Input: part model. Units: mm. Frame: model coordinates. A direction names the side the tool comes from. Give positions to 0.01 mm unless a question says otherwise; leave off trailing zeros. Write each loop counter-clockwise with the first axis right and the second up, starting at its lowest first coordinate (ties: lowest second). Pieces come first, ordered by that corner, then holes. Notation, with made-up numbers: (-14, 88.5) -> (8, 88.5) arc R20 cw to (8, 105.5) -> close; hole circle Ø4 at (-25, 57.25). An arc over 180 degrees is marked (long way). Return JSON: item names as keys, results as strings. Group by question number.
Item 1: Section C-C, the plane y = 7. Return loops of the section in (x, z) (3 decimals).
Item 2: Pin query (flat end, axial travel): P1, Ø5, axis at x = 17.5, z = -1.5, coming from the -Y side; P2, Ø5, axis at x = 17.5, z = 7.5, coming from the +Y side. Return the tip coordinate at first contact, or that it passes through.
Item 3: Set-up query: faces 1 (the face through (11.4, 3.94, 3.93)), 2 (the face through (0, 8, -6)). Return all of +Z, -Z, +X, -X, +Y, -Y with unobstructed straight access to the full face (end or side cutting, diameter ignored); none if empty.
Item 4: Section B-B, the plane z = 1. Return loops of the section in (x, y).
Item 5: Section D-D, the plane x = -17.5. Return loops of the section in (y, z) (3 decimals).
Item 6: Mould query, pull axis X, two halves, no side actions, for faces 3 (the face through (22.5, 4, 0)), 4 (the face through (0, 4, -12.5)), 5 (the face through (-11.4, 3.94, -3.93)). Classes: released by +X, released by -X, zero draft, split by the parting line, or undercut.
Item 7: Section A-A, the plane z = 7.5. Return loops of the section in (x, y) (3 decimals), then the cut area to 3 significant figures.
Item 8: Line query: line 1 (X direction, y = 5.5, z = -7.5); line 2 (X direction, y = 0.5, z = 7.25); line 3 (Z direction, x = 0, y = 4). Output: solid intervals per line, ascending. Write a range as [from, to].
from build123d import *

# Parameters (mm, degrees)
SKETCH_1_W          = 45
SKETCH_1_H          = 25
EXTRUDE_1_DEPTH     = 8
SKETCH_2_R          = 2.15
SKETCH_2_R_2        = 3.175
CUT_EXTRUDE_1_DEPTH = 27.953663944
SKETCH_3_W          = 24
SKETCH_3_H          = 9
CUT_EXTRUDE_2_DEPTH = 27.953663944
FILLET_1_R          = 2


with BuildPart() as part:
    # 草图1 → 凸台-拉伸1 (new body)
    with BuildSketch(Plane(origin=(0, 0, 0), x_dir=(1, 0, 0), z_dir=(0, 1, 0))):
        Rectangle(SKETCH_1_W, SKETCH_1_H)
    extrude(amount=EXTRUDE_1_DEPTH)

    # 草图2 → 切除-拉伸1 (cut, through all)
    with BuildSketch(Plane(origin=(0, 8, 0), x_dir=(1, 0, 0), z_dir=(0, 1, 0))):
        with Locations(Location((-17.5, 7.5, 0), (0, 0, 270))):
            Circle(SKETCH_2_R)
        with Locations(Location((17.5, 7.5, 0), (0, 0, 270))):
            Circle(SKETCH_2_R)
        with Locations(Location((17.5, -7.5, 0), (0, 0, 270))):
            Circle(SKETCH_2_R_2)
        with Locations(Location((-17.5, -7.5, 0), (0, 0, 270))):
            Circle(SKETCH_2_R_2)
    extrude(amount=-CUT_EXTRUDE_1_DEPTH, mode=Mode.SUBTRACT)

    # 草图3 → 切除-拉伸2 (cut, through all)
    with BuildSketch(Plane(origin=(0, 8, 0), x_dir=(1, 0, 0), z_dir=(0, 1, 0))):
        Rectangle(SKETCH_3_W, SKETCH_3_H)
    extrude(amount=-CUT_EXTRUDE_2_DEPTH, mode=Mode.SUBTRACT)

    # 圆角1
    fillet_1_edges = [part.edges().sort_by_distance(p)[0] for p in [
        (-12, 4, 4.5),
        (-12, 4, -4.5),
        (12, 4, -4.5),
        (12, 4, 4.5),
    ]]
    fillet(fillet_1_edges, radius=FILLET_1_R)


solid = part.part
Answer below:
{
 "1": {"outline": "(-22.5, -12.5) -> (22.5, -12.5) -> (22.5, 12.5) -> (-22.5, 12.5) -> close; hole circle Ø6.35 at (-17.5, 7.5); hole circle Ø4.3 at (-17.5, -7.5); hole (-12, -2.5) arc R2 ccw to (-10, -4.5) -> (10, -4.5) arc R2 ccw to (12, -2.5) -> (12, 2.5) arc R2 ccw to (10, 4.5) -> (-10, 4.5) arc R2 ccw to (-12, 2.5) -> close; hole circle Ø6.35 at (17.5, 7.5); hole circle Ø4.3 at (17.5, -7.5)"},
 "2": {"P1": "stops at y = 0", "P2": "passes through"},
 "3": {"face 1": "+Y, -Y", "face 2": "+Z, -Z, +X, -X, +Y"},
 "4": {"outline": "(-22.5, 0) -> (-12, 0) -> (-12, 8) -> (-22.5, 8) -> close; (12, 0) -> (22.5, 0) -> (22.5, 8) -> (12, 8) -> close"},
 "5": {"outline": "(0, -12.5) -> (8, -12.5) -> (8, -9.65) -> (0, -9.65) -> close; (0, -5.35) -> (8, -5.35) -> (8, 4.325) -> (0, 4.325) -> close; (0, 10.675) -> (8, 10.675) -> (8, 12.5) -> (0, 12.5) -> close"},
 "6": {"face 3": "released by +X", "face 4": "zero draft", "face 5": "undercut"},
 "7": {"outline": "(-22.5, 0) -> (-20.675, 0) -> (-20.675, 8) -> (-22.5, 8) -> close; (-14.325, 0) -> (14.325, 0) -> (14.325, 8) -> (-14.325, 8) -> close; (20.675, 0) -> (22.5, 0) -> (22.5, 8) -> (20.675, 8) -> close", "area": "258 mm2"},
 "8": {"line 1": "x = [-22.5, -19.65], [-15.35, 15.35], [19.65, 22.5]", "line 2": "x = [-22.5, -20.67], [-14.33, 14.33], [20.67, 22.5]", "line 3": "z = [-12.5, -4.5], [4.5, 12.5]"}
}
